The model under review builds one solid part; all positions refer to its coordinate system, in mm. Face numbers are marked on the shaded views. A direction names the side the tool comes from. Give positions to 0.01 mm unless a question says otherwise; leave off trailing zeros. Order: outer loops, then holes, each group sorted by start corner. A loop starts at its lowest first (then second) coordinate and runs counter-clockwise, first axis right, second up. Notation, with made-up numbers: (63.5, 89.25) - (99.5, 89.25) arc R17 cw to (99.5, 113.25) - close; hole circle Ø10 at (81.5, -12.5). An arc over 180 degrees is marked (long way). Write item = value, one per line. Start each with the question number.
1. For P1, Ø3, axis at x = 18.1, y = 18.1, coming from the -Z side; P2, Ø15, axis at y = 18, z = 19, coming from the +X side; P3, Ø2, axis at y = 18.1, z = 19.6, coming from the +X side; P4, Ø15, axis at x = 12, z = 14, coming from the +Y side, all flat-tipped, find the tip position at first contact; note any pin that passes through.
2. We need section C-C, the plane z = 28.5. Give the boundary of the cut face in (x, y).
3. Mouldability with a two-part tool opening along X and no side actions: class the marked faces 5, 6 and 7 as pulls with the +X half, pulls with the -X half, needs draft (parallel to the pull), parting line crosses it, or undercut.
4. Wall thickness on probe 1 along X at (y, z) = (24, 26); probe 2 along X at (y, z) = (18.1, 0.65): over which ranges is each line inside the solid? List them lowest first.
5. We need section A-A, the plane y = 18.1. State how many separate pieces and enclosed holes the cut face has, and give its area (3 significant figures).
6. Machinability: for the marked faces 1, 2, 3 and 4, which of the approach directions +Z, -Z, +X, -X, +Y, -Y give a long, thin tool a straight path to every point of the face, cutting with its end or side? Answer none if there is none.
from build123d import *

# Parameters (mm, degrees)
F0_W           = 56.2
F0_H           = 56.2
F1_DEPTH       = 3
F2_W           = 36.2
F2_H           = 36.2
F2_W_2         = 30.2
F2_H_2         = 30.2
F3_DEPTH       = 33.2
F4_D           = 3.5
F4_DEPTH       = 13.5
F4_CSINK_D     = 7.2
F4_CSINK_ANGLE = 90
F4_TIP         = 1.0515060833
F5_R           = 1.49999
F7_D           = 3.5
F7_DEPTH       = 13.5
F7_CSINK_D     = 7.2
F7_CSINK_ANGLE = 90
F7_TIP         = 1.0515060833


# Not quite as in the source:
# - a fillet or chamfer is up to 0.001 mm smaller than in the source, because OpenCascade refuses the exact size
# - a feature names something its author has since deleted; it is built from what else it names


with BuildPart() as f1:
    # F0 (on Top) → F1 (new body)
    with BuildSketch(Plane.XY):
        with Locations((18.1, 18.1)):
            Rectangle(F0_W, F0_H)
    extrude(amount=F1_DEPTH)

    # F2 (on face) → F3 (join)
    with BuildSketch(Plane.XY.offset(3)):
        with Locations((18.1, 18.1)):
            Rectangle(F2_W, F2_H)
        with Locations((18.1, 18.1)):
            Rectangle(F2_W_2, F2_H_2, mode=Mode.SUBTRACT)
    extrude(amount=F3_DEPTH)

    # F4
    with Locations(Plane.XY.offset(3)):
        with Locations((18.1, 18.1)):
            CounterSinkHole(F4_D / 2, F4_CSINK_D / 2, depth=F4_DEPTH, counter_sink_angle=F4_CSINK_ANGLE)
            with Locations((0, 0, -(F4_DEPTH + F4_TIP / 2))):  # 118° drill point
                Cone(0, F4_D / 2, F4_TIP, mode=Mode.SUBTRACT)

    # F5 (radius 1.5 in the source; OpenCascade refuses exactly that, so slightly less here)
    f5_edges = [f1.edges().sort_by_distance(p)[0] for p in [
        (33.2, 18.1, 36.2),
        (18.1, 3, 36.2),
        (18.1, 0, 3),
        (18.1, 33.2, 36.2),
        (3, 18.1, 36.2),
        (0, 18.1, 36.2),
        (18.1, 36.2, 36.2),
        (36.2, 18.1, 36.2),
        (18.1, 0, 36.2),
        (36.2, 0, 19.6),
        (0, 0, 19.6),
        (0, 18.1, 3),
        (18.1, 36.2, 3),
        (36.2, 36.2, 19.6),
        (0, 36.2, 19.6),
        (18.1, 46.2, 3),
        (-10, 18.1, 3),
        (18.1, -10, 3),
        (46.2, 18.1, 3),
        (36.2, 18.1, 3),
    ]]
    fillet(f5_edges, radius=F5_R)

    # F7
    with Locations(Plane.YZ.offset(36.2)):
        with Locations((18.1, 19.6)):
            CounterSinkHole(F7_D / 2, F7_CSINK_D / 2, depth=F7_DEPTH, counter_sink_angle=F7_CSINK_ANGLE)
            with Locations((0, 0, -(F7_DEPTH + F7_TIP / 2))):  # 118° drill point
                Cone(0, F7_D / 2, F7_TIP, mode=Mode.SUBTRACT)


solid = f1.part
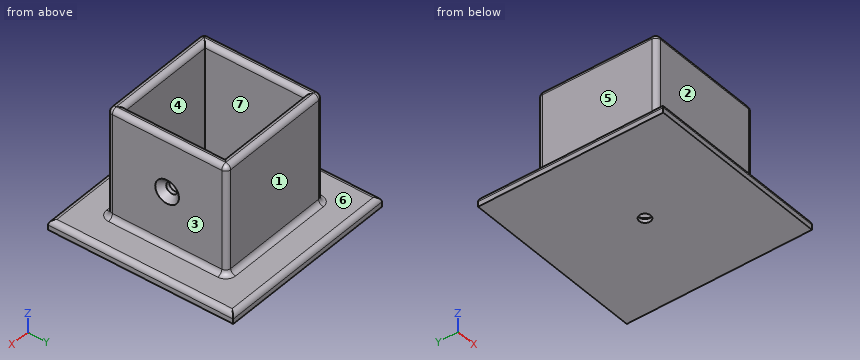
Model answer:
q1.P1 = through
q1.P2 = 36.2
q1.P3 = 3
q1.P4 = 36.2
q2.outline = (0, 1.5) arc R1.5 ccw to (1.5, 0) - (34.7, 0) arc R1.5 ccw to (36.2, 1.5) - (36.2, 34.7) arc R1.5 ccw to (34.7, 36.2) - (1.5, 36.2) arc R1.5 ccw to (0, 34.7) - close; hole (3, 3) - (33.2, 3) - (33.2, 33.2) - (3, 33.2) - close
q3.face_5 = pulls with the -X half
q3.face_6 = needs draft
q3.face_7 = undercut
q4.probe_1 = 0 to 3, 33.2 to 36.2
q4.probe_2 = -10 to 16.35, 19.85 to 46.2
q5.separate_pieces = 3
q5.enclosed_holes = 0
q5.area = 338 mm2
q6.face_1 = +Z, +X, -X, +Y
q6.face_2 = +Z, +X, -X, -Y
q6.face_3 = +Z, +X, +Y, -Y
q6.face_4 = +Z
